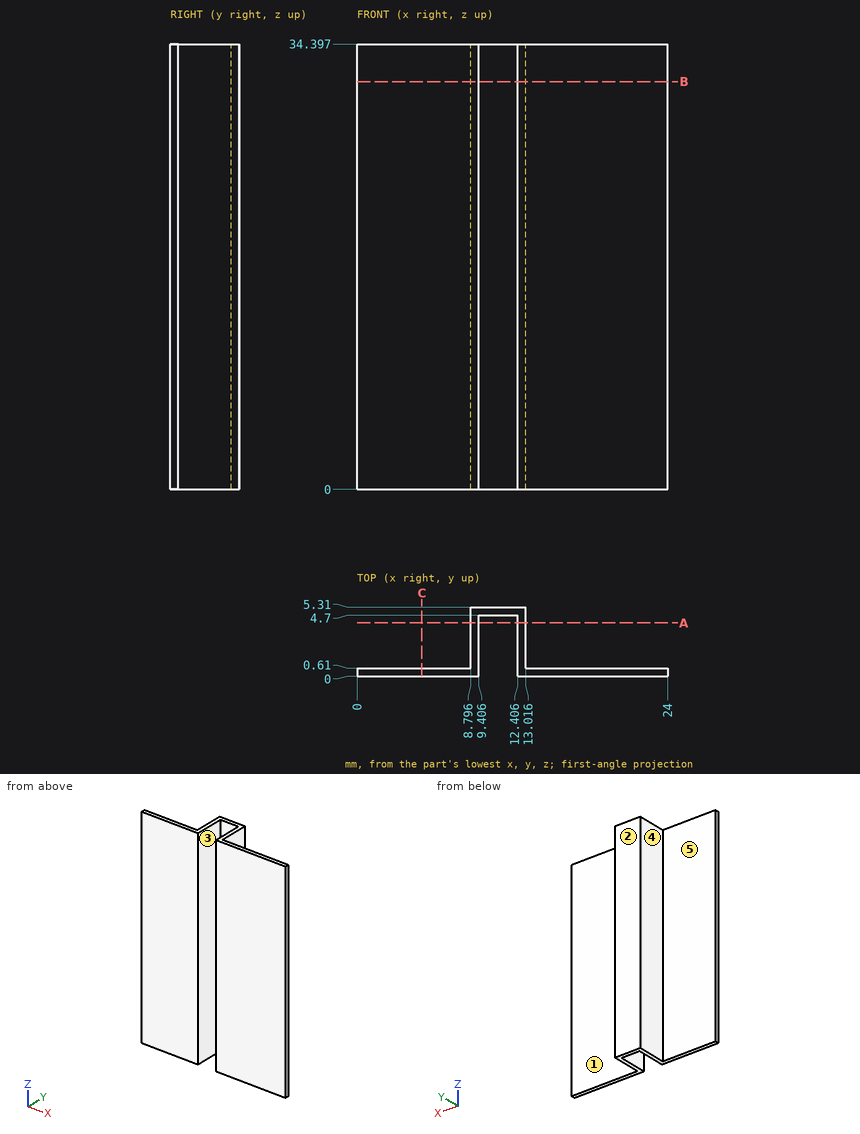
Design review of the part shown in the three views and the two pictorial views. Dimensions are in mm from the part's minimum x, y and z. A direction names the side the tool comes from. Give positions to 0.01 mm unless a question says otherwise; leave off trailing zeros. Write each loop counter-clockwise with the first axis right and the second up, starting at its lowest first coordinate (ties: lowest second). Pieces come first, ordered by that corner, then holes.
(1) Add section A-A (y = 4.1). Give the boundary of the cut face in (x, z) (1 decimal).
Checked values:
outline: (8.8, 0) - (9.4, 0) - (9.4, 34.4) - (8.8, 34.4) - close; (12.4, 0) - (13, 0) - (13, 34.4) - (12.4, 34.4) - close
(2) Wall thickness on line 1 along X through (y, z) = (2.9, 32) (1 decimal); line 2 along X through (y, z) = (0.3, 30.5) (1 decimal); line 3 along Y through (x, z) = (18.25, 3): over which ranges is each line inside the solid? List them lowest first.
Checked values:
line 1: x = 8.8 to 9.4, 12.4 to 13
line 2: x = 0 to 9.4, 12.4 to 24
line 3: y = 0 to 0.61
(3) Clearance check with flat-ended pins moving along their axes: pin 1 Ø1.4 at (y, z) = (1.5, 23) entering from -X (1 decimal); pin 2 Ø2 at (x, y) = (20.5, 3.5) entering from +Z; pin 3 Ø4.5 at (x, z) = (6.5, 18.5) entering from +Y. State where each tip first meets the part, or that it passes through.
Checked values:
pin 1: stops at x = 8.8
pin 2: passes through
pin 3: stops at y = 0.61
(4) Tool access review of the marked faces 1 and 2: name each direction out of +Z, -Z, +X, -X, +Y, -Y from which nothing blocks a thin tool from reaching the whole face with its end or side.
Checked values:
face 1: +Z, -Z, +X, +Y
face 2: +Z, -Z, +X, -X, +Y
(5) Add section B-B (z = 31.5). Give the boundary of the cut face in (x, y) (1 decimal).
Checked values:
outline: (0, 0) - (9.4, 0) - (9.4, 4.7) - (12.4, 4.7) - (12.4, 0) - (24, 0) - (24, 0.6) - (13, 0.6) - (13, 5.3) - (8.8, 5.3) - (8.8, 0.6) - (0, 0.6) - close
(6) Add section C-C (x = 5). Give the boundary of the cut face in (y, z).
Checked values:
outline: (0, 0) - (0.61, 0) - (0.61, 34.4) - (0, 34.4) - close
(7) Mouldability with a two-part tool opening along X and no side actions: class the marked faces 3, 4 and 5 as +X half, -X half, draft (parallel to the pull), parting line (faces both ways), or undercut.
Checked values:
face 3: undercut
face 4: -X half
face 5: draft
